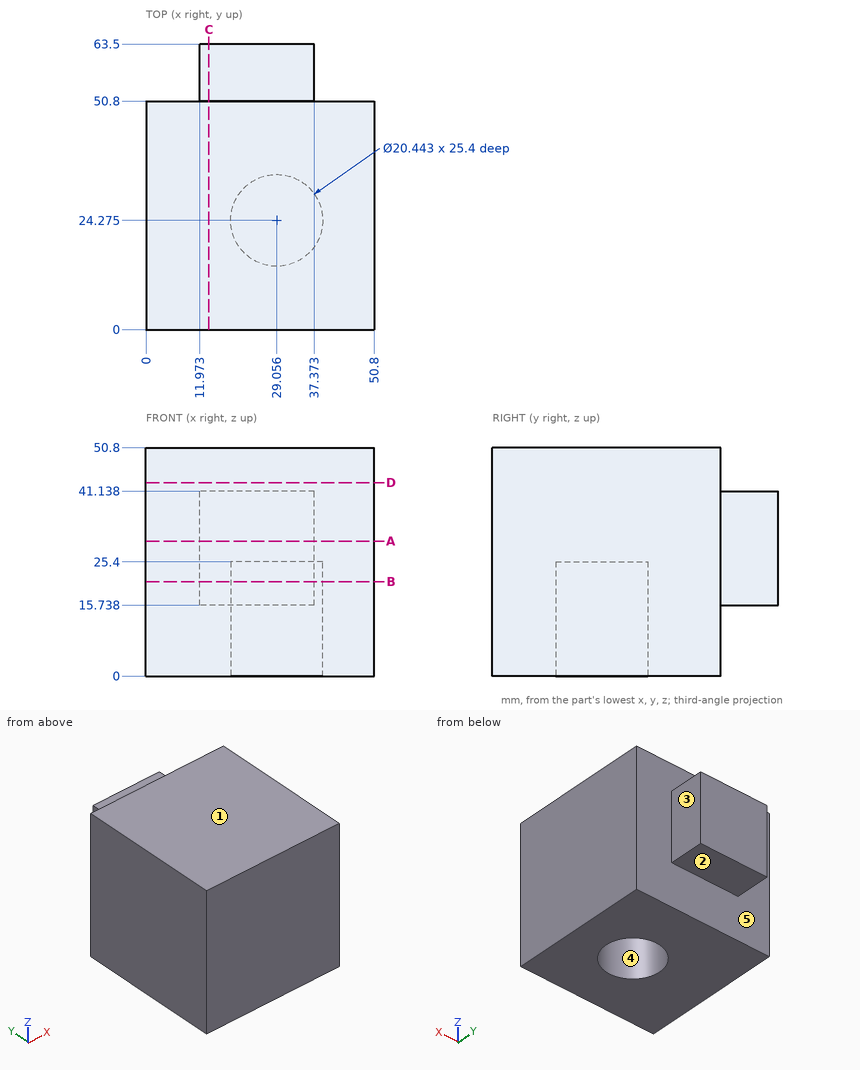
Could you check a few things on this drawing? It's one solid part, dimensions in mm from its lowest x, y, z. A direction names the side the tool comes from. Round coordinates to 2 decimals unless told otherwise and drop trailing zeros. Write each loop counter-clockwise with the first axis right and the second up, starting at its lowest first coordinate (ties: lowest second). Pieces come first, ordered by that corner, then holes. Notation, with made-up numbers: (13.5, -16) -> (22.5, -16) arc R9 cw to (22.5, -4) -> close; hole circle Ø7 at (10.5, 62). An arc over 180 degrees is marked (long way). One line per item, written item: value.
1) Suppose I cut it at D-D on z = 43. List the corners of the cut face in (x, y) for me.
Filled sheet:
outline: (0, 0) -> (50.8, 0) -> (50.8, 50.8) -> (0, 50.8) -> close
2) I'm going to push flat-ended pins straight in: pin 1 Ø14 at (x, y) = (21.5, 59) entering from -Z; pin 2 Ø10 at (y, z) = (58.5, 28) entering from -X; pin 3 Ø5 at (x, z) = (44.5, 20.5) entering from +Y; pin 4 Ø12 at (x, y) = (44, 57) entering from -Z. Where does each tip first touch, or does it pass through?
Filled sheet:
pin 1: stops at z = 15.74
pin 2: stops at x = 11.97
pin 3: stops at y = 50.8
pin 4: passes through
3) Suppose I cut it at A-A on z = 30. List the corners of the cut face in (x, y) for me, plus the area to 3 significant figures.
Filled sheet:
outline: (0, 0) -> (50.8, 0) -> (50.8, 50.8) -> (37.37, 50.8) -> (37.37, 63.5) -> (11.97, 63.5) -> (11.97, 50.8) -> (0, 50.8) -> close
area: 2,900 mm2
4) If I drill on line 1 (X direction, y = 51.5, z = 22); line 2 (Y direction, x = 10, z = 31); line 3 (Y direction, x = 20.5, z = 14) (1 decimal), over which ranges is the centre line in solid material (lowest first)? Write a range as [from, to].
Filled sheet:
line 1: x = [11.97, 37.37]
line 2: y = [0, 50.8]
line 3: y = [0, 18.7], [29.9, 50.8]
5) Suppose I cut it at B-B on z = 21. List the corners of the cut face in (x, y) for me (1 decimal), plus the area to 4 significant figures.
Filled sheet:
outline: (0, 0) -> (50.8, 0) -> (50.8, 50.8) -> (37.4, 50.8) -> (37.4, 63.5) -> (12, 63.5) -> (12, 50.8) -> (0, 50.8) -> close; hole circle Ø20.4 at (29.1, 24.3)
area: 2,575 mm2
6) For the marked faces 1 and 2, which set-ups out of +Z, -Z, +X, -X, +Y, -Y let a thin tool reach every point of the face, with its end or its side?
Filled sheet:
face 1: +Z, +X, -X, +Y, -Y
face 2: -Z, +X, -X, +Y
7) Suppose I cut it at C-C on x = 14. List the corners of the cut face in (y, z) for me.
Filled sheet:
outline: (0, 0) -> (50.8, 0) -> (50.8, 15.74) -> (63.5, 15.74) -> (63.5, 41.14) -> (50.8, 41.14) -> (50.8, 50.8) -> (0, 50.8) -> close
8) We'd pull the mould along X, two halves only. Please class the marked faces 3, 4 and 5: released by +X, released by -X, zero draft, split by the parting line, or undercut.
Filled sheet:
face 3: released by +X
face 4: undercut
face 5: zero draft
